Part model, mm, in its own coordinate system. Round coordinates to 2 decimals unless told otherwise and drop trailing zeros. Loops run counter-clockwise (first coordinate to the right, second up) from the corner with the lowest first, then second, coordinate; pieces in that order, holes last. Notation, with made-up numbers: M 35.5,74.25 L 84.5,74.25 A23 ccw 84.5,98.25 Z; hole C 79.25,-29 d1. An arc over 180 degrees is marked long. Put each result on its own line as item: value. Start each with the question number.
1) Slice it at C-C on z = 1.1. Give the cut face in (x, y) (3 decimals), then the cut area to 3 significant figures.
2) Slice it at D-D on x = 15. Give the cut face in (y, z).
3) Probe line 1 along X through (y, z) = (7.5, 0.15); line 2 along X through (y, z) = (8, 0.65); line 3 along Y through (x, z) = (11.5, 1.35). List the from-to ranges inside material, lowest first.
4) Slice it at A-A on x = 4.94. Give the cut face in (y, z), then the cut area to 3 significant figures.
5) Slice it at B-B on y = 16.5. Give the cut face in (x, z).
6) Pull direction X, two halves, no side cores. Call faces 1 (the flat face through (1, 2, 0)), 2 (the cylindrical face through (-15.64, -18.6, 0.99)), 3 (the cylindrical face through (-0.595, -8.558, 0.986)): +X half, -X half, draft (parallel to the pull), parting line (faces both ways), or undercut.
```python
from build123d import *

# Parameters (mm, degrees)
SKETCH_2_W              = 37
SKETCH_2_H              = 39
EXTRUDE_1_DEPTH         = 2
SKETCH_3_R              = 1.75
CUT_EXTRUDE_2_DEPTH     = 2
CHAMFER_3_SIZE          = 1
SKETCH_7_R              = 4.25
CUT_EXTRUDE_3_DEPTH     = 10
SKETCH_8_W              = 2
SKETCH_8_H              = 39
CUT_EXTRUDE_4_DEPTH     = 10
FILLET_3_R              = 3
M2_5_TAPPED_HOLE1_D     = 2.05
M2_5_TAPPED_HOLE1_DEPTH = 7.25
M2_5_TAPPED_HOLE1_TIP   = 0.615882135
CHAMFER2_SIZE           = 4
SKETCH_9_W              = 35
SKETCH_9_H              = 2
EXTRUDE_1_2_DEPTH       = 5
CHAMFER_5_SIZE          = 4
FILLET_4_R              = 10
SKETCH_11_R             = 5
CUT_EXTRUDE_1_DEPTH     = 31.765240126


with BuildPart() as part:
    # 草图2 → Extrude 1 (new body)
    with BuildSketch(Plane.XY):
        Rectangle(SKETCH_2_W, SKETCH_2_H)
    extrude(amount=EXTRUDE_1_DEPTH)

    # 草图3 → 拉伸2 (cut)
    with BuildSketch(Plane.XY.offset(2)):
        with Locations((-13.5, 16.5)):
            Circle(SKETCH_3_R)
        with Locations((-13.5, -16.5)):
            Circle(SKETCH_3_R)
    extrude(amount=-CUT_EXTRUDE_2_DEPTH, mode=Mode.SUBTRACT)

    # 倒角3
    chamfer_3_edges = [part.edges().sort_by_distance(p)[0] for p in [
        (-18.5, 19.5, 1),
        (-18.5, -19.5, 1),
    ]]
    chamfer(chamfer_3_edges, length=CHAMFER_3_SIZE)

    # 草图7 → 拉伸3 (cut)
    with BuildSketch(Plane.XY.offset(2)):
        with Locations((4.94, 0)):
            Circle(SKETCH_7_R)
    extrude(amount=-CUT_EXTRUDE_3_DEPTH, mode=Mode.SUBTRACT)

    # 草图8 → 拉伸4 (cut)
    with BuildSketch(Plane.XY.offset(2)):
        with Locations((-17.5, 0)):
            Rectangle(SKETCH_8_W, SKETCH_8_H)
    extrude(amount=-CUT_EXTRUDE_4_DEPTH, mode=Mode.SUBTRACT)

    # 圆角3
    fillet_3_edges = [part.edges().sort_by_distance(p)[0] for p in [
        (-16.5, -19.5, 1),
    ]]
    fillet(fillet_3_edges, radius=FILLET_3_R)

    # M2.5 Tapped Hole1
    with Locations(Plane(origin=(-0.816889803, -7.556998068, 2), x_dir=(1, 0, 0), z_dir=(0, 0, 1))):
        with Locations((0, 0), (11.513779606, 15.113996136), (0, 15.113996136), (11.513779606, 0)):
            Hole(M2_5_TAPPED_HOLE1_D / 2, depth=M2_5_TAPPED_HOLE1_DEPTH)
            with Locations((0, 0, -(M2_5_TAPPED_HOLE1_DEPTH + M2_5_TAPPED_HOLE1_TIP / 2))):  # 118° drill point
                Cone(0, M2_5_TAPPED_HOLE1_D / 2, M2_5_TAPPED_HOLE1_TIP, mode=Mode.SUBTRACT)

    # Chamfer2
    chamfer2_edges = [part.edges().sort_by_distance(p)[0] for p in [
        (18.5, -19.5, 1),
    ]]
    chamfer(chamfer2_edges, length=CHAMFER2_SIZE)

    # 草图9 → Extrude 1 2 (add)
    with BuildSketch(Plane(origin=(0, 19.5, 0), x_dir=(1, 0, 0), z_dir=(0, 1, 0))):
        with Locations((1, -1)):
            Rectangle(SKETCH_9_W, SKETCH_9_H)
    extrude(amount=EXTRUDE_1_2_DEPTH)

    # 倒角5
    chamfer_5_edges = [part.edges().sort_by_distance(p)[0] for p in [
        (18.5, 24.5, 1),
    ]]
    chamfer(chamfer_5_edges, length=CHAMFER_5_SIZE)

    # 圆角4
    fillet_4_edges = [part.edges().sort_by_distance(p)[0] for p in [
        (-16.5, 24.5, 1),
    ]]
    fillet(fillet_4_edges, radius=FILLET_4_R)

    # 草图11 → 切除-拉伸1 (cut, through all)
    with BuildSketch(Plane.XY.offset(2)):
        with Locations((-1.5, 24.5)):
            Circle(SKETCH_11_R)
    extrude(amount=-CUT_EXTRUDE_1_DEPTH, mode=Mode.SUBTRACT)


solid = part.part
```
Recorded:
1. outline: M -16.5,-16.5 A3 ccw -13.5,-19.5 L 14.5,-19.5 L 18.5,-15.5 L 18.5,20.5 L 14.5,24.5 L 3.5,24.5 A5 cw -6.5,24.5 A10 ccw -16.5,14.5 Z; hole C -13.5,-16.5 d3.5; hole C -13.5,16.5 d3.5; hole C -0.817,-7.557 d2.05; hole C -0.817,7.557 d2.05; hole C 4.94,0 d8.5; hole C 10.697,-7.557 d2.05; hole C 10.697,7.557 d2.05
1. area: 1,370 mm2
2. outline: M -19,0 L 24,0 L 24,2 L -19,2 Z
3. line 1: x = -16.5 to -1.84, 0.21 to 9.67, 11.72 to 18.5
3. line 2: x = -16.5 to -1.74, 0.11 to 9.77, 11.62 to 18.5
3. line 3: y = -19.5 to -8.19, -6.92 to 6.92, 8.19 to 24.5
4. outline: M -19.5,0 L -4.25,0 L -4.25,2 L -19.5,2 Z; M 4.25,0 L 24.5,0 L 24.5,2 L 4.25,2 Z
4. area: 71.0 mm2
5. outline: M -16.3,0 L -15.25,0 L -15.25,2 L -16.3,2 Z; M -11.75,0 L 18.5,0 L 18.5,2 L -11.75,2 Z
6. face 1: draft
6. face 2: -X half
6. face 3: undercut
